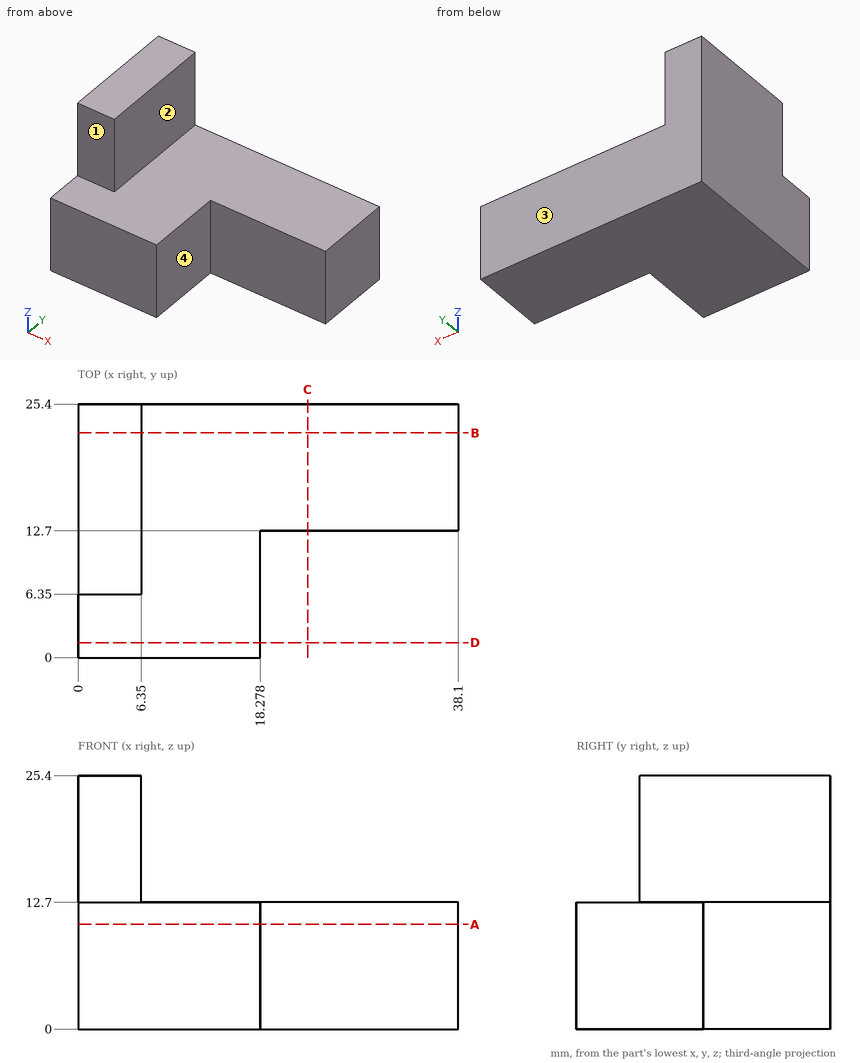
Input: dimensioned drawing with shaded views. Units: mm. Origin: part minimum x, y, z. A direction names the side the tool comes from. Round coordinates to 2 decimals unless told otherwise and drop trailing zeros. Loops run counter-clockwise (first coordinate to the right, second up) from the corner with the lowest first, then second, coordinate; pieces in that order, holes last. Notation, with made-up numbers: M 3.25,-34.5 L 55.25,-34.5 A35 ccw 55.25,4.5 Z; hole C 85.25,71 d1. An arc over 180 degrees is marked long. One line per question, with ' | ' between items.
(1) Cut plane B-B on y = 22.5. Return the cut outline in (x, z).
Check result:
outline: M 0,0 L 38.1,0 L 38.1,12.7 L 6.35,12.7 L 6.35,25.4 L 0,25.4 Z
(2) Access query for the marked faces 1, 2, 3 and 4. Directions: +Z, -Z, +X, -X, +Y, -Y. A direction counts if a zero-diameter tool reaches every point of the face in a straight line with its end or side. Return the directions, or none.
Check result:
face 1: +Z, +X, -X, -Y | face 2: +Z, +X, +Y, -Y | face 3: +Z, -Z, +X, -X, +Y | face 4: +Z, -Z, +X, -Y
(3) Cut plane D-D on y = 1.5. Return the cut outline in (x, z).
Check result:
outline: M 0,0 L 18.28,0 L 18.28,12.7 L 0,12.7 Z
(4) Contact query for flat-ended pins moving along their axis: P1, Ø4, axis at y = 11.5, z = 19, coming from the +X side; P2, Ø5, axis at x = 8.5, y = 14, coming from the +Z side; P3, Ø12, axis at x = 33.5, y = 17, coming from the +Z side; P4, Ø14, axis at x = 26.5, z = 7.5, coming from the -Y side. Output: stop coordinate, or through.
Check result:
P1: stops at x = 6.35 | P2: stops at z = 25.4 | P3: stops at z = 12.7 | P4: stops at y = 12.7
(5) Material intervals for line 1 along X through (y, z) = (7.25, 15.5); line 2 along X through (y, z) = (6.25, 2); line 3 along Z through (x, y) = (8.5, 7.5), sorted ascending. Write a range as from..to.
Check result:
line 1: x = 0..6.35 | line 2: x = 0..18.28 | line 3: z = 0..12.7
(6) Cut plane A-A on z = 10.5. Return the cut outline in (x, y), plus the area to 3 significant figures.
Check result:
outline: M 0,0 L 18.28,0 L 18.28,12.7 L 38.1,12.7 L 38.1,25.4 L 0,25.4 Z | area: 716 mm2
(7) Cut plane C-C on x = 23. Return the cut outline in (y, z).
Check result:
outline: M 12.7,0 L 25.4,0 L 25.4,12.7 L 12.7,12.7 Z
